Autodesk Inventor part; units mm, degrees
ref_plane "YZ Plane" through (0, 0, 0) normal (1, 0, 0) x (0, 1, 0)
ref_plane "XZ Plane" through (0, 0, 0) normal (0, 1, 0) x (-1, 0, 0)
ref_plane "XY Plane" through (0, 0, 0) normal (0, 0, 1) x (1, 0, 0)
sketch "Sketch1" plane through (0, 0, 0) normal (1, 0, 0) x (0, 1, 0)
  line L0 (0, 0) -> (5.55, 0)
  line L1 (5.55, 0) -> (5.55, 5.6)
  line L2 (5.55, 5.6) -> (20.55, 5.6)
  line L3 (20.55, 5.6) -> (20.55, 2.4)
  line L4 (20.55, 2.4) -> (10.05, 2.4)
  line L5 (10.05, 2.4) -> (10.05, 4)
  line L6 (10.05, 4) -> (7.55, 4)
  line L7 (7.55, 4) -> (7.55, -29)
  line L8 (0, 0) -> (0, -29)
  line L9 (0, -29) -> (7.55, -29)
  dimension "d1" = 5.55
  dimension "d2" = 15
  dimension "d3" = 2
  dimension "d4" = 2.5
  dimension "d5" = 1.6
  dimension "d6" = 29
  dimension "d7" = 33
  dimension "d8" = 3.2
extrude "Extrusion1" add sketch "Sketch1" along normal blind 18
sketch "Sketch2" plane through (0, 10.05, 2.4) normal (0, 0, -1) x (-1, 0, 0)
  line L0 (0, 0) -> (-18, 0)
  line L1 (-9, 0) -> (-9, -5.1044) construction
  line L2 (-13, 2.82) -> (-5, 2.82)
  line L3 (-5, 2.82) -> (-5, -0.28)
  line L4 (-5, -0.28) -> (-13, -0.28)
  line L5 (-13, -0.28) -> (-13, 2.82)
  point P0 (0, -10.05)
  point P1 (-9, -0.28)
  dimension "d11" = 3.1
  dimension "d12" = 8
extrude "Extrusion2" cut sketch "Sketch2" against normal up to surface (3.2 mm away)
chamfer "Chamfer1" distance 1.2 angle 45 2 edges at (5, 9.77, 4.8) (13, 9.77, 4.8)
chamfer "Chamfer2" distance 1.6 angle 45 2 edges at (15.04, 10.05, 2.4) (2.96, 10.05, 2.4)
fillet "Fillet1" radius 1 4 edges at (9, 5.55, 5.6) (9, 20.55, 5.6) (18, 13.05, 5.6) (0, 13.05, 5.6)
sketch "Sketch3" plane through (0, 0, -29) normal (0, 0, -1) x (-1, 0, 0)
  line L0 (0, 7.55) -> (-18, 7.55)
  line L1 (-9, 7.55) -> (-9, 5.1292) construction
  line L2 (-18, 7.55) -> (-15, 7.55)
  line L3 (-15, 7.55) -> (-15, 5.95)
  line L4 (-15, 5.95) -> (-18, 5.95)
  line L5 (-18, 5.95) -> (-18, 7.55)
  line L6 (0, 7.55) -> (-3, 7.55)
  line L7 (-3, 7.55) -> (-3, 5.95)
  line L8 (-3, 5.95) -> (0, 5.95)
  line L9 (0, 5.95) -> (0, 7.55)
  line L10 (0, 7.55) -> (-18, 7.55)
  line L11 (-18, 0) -> (-18, 7.55)
  point P0 (0, 0)
  dimension "d22" = 3
  dimension "d23" = 1.6
extrude "Extrusion3" cut sketch "Sketch3" against normal up to surface (33 mm away)
chamfer "Chamfer3" distance 1.6 angle 45 2 edges at (16.5, 5.95, 4) (1.5, 5.95, 4)
sketch "Sketch4" plane through (0, 0, 0) normal (-1, 0, 0) x (0, 0, 1)
  line L0 (-17, 0) -> (-7, 0)
  line L1 (-7, 0) -> (-7, 16.55)
  line L2 (-7, 16.55) -> (-17, 16.55)
  line L3 (-17, 16.55) -> (-17, 0)
  line L4 (2.4, 5.95) -> (-29, 5.95)
  line L5 (-29, 0) -> (0, 0)
  line L6 (0, 0) -> (0, 5.55)
  line L7 (4.6, 20.55) -> (2.4, 20.55)
  dimension "d29" = 10
  dimension "d30" = 7
  dimension "d31" = 4
extrude "Extrusion4" add sketch "Sketch4" along normal blind 5
sketch "Sketch5" plane through (0, 16.55, -7) normal (0, 1, 0) x (1, 0, 0)
  line L0 (0, -9.4) -> (18, -9.4)
  line L1 (0, 0) -> (-5, 0)
  line L2 (0, 0) -> (0, 10)
  line L3 (0, 10) -> (-5, 10)
  line L4 (-5, 0) -> (-5, 10)
  line L5 (0, 10) -> (0, 22)
  line L6 (-5, 10) -> (-5, 0)
  line L7 (0, 10) -> (-5, 10)
  line L8 (-5, 10) -> (-5, 0)
  line L9 (-5, 0) -> (0, 0)
  line L10 (13, -9.4) -> (5, -9.4)
  line L11 (13, -9.4) -> (18, -9.4)
  line L12 (5, -9.4) -> (18, -9.4)
  line L13 (18, -9.4) -> (0, 10)
  line L14 (3, -9.4) -> (0, -9.4)
  line L15 (0, 0) -> (0, -9.4)
  line L16 (0, -9.4) -> (18, -9.4)
  point P0 (0, -7)
extrude "Extrusion5" add sketch "Sketch5" against normal blind 2.5
chamfer "Chamfer4" distance 1.35 angle 45 3 edges at (-5, 8.275, -7) (-5, 8.275, -17) (0, 2.975, -17)
properties part number "pro_micro_mount"
Geometry: final body of the model. Coordinates: model frame, mm. A direction names the side the tool comes from. Round coordinates to 2 decimals unless told otherwise and drop trailing zeros. Write each loop counter-clockwise with the first axis right and the second up, starting at its lowest first coordinate (ties: lowest second). Pieces come first, ordered by that corner, then holes.
Item 1: Section query D-D (z = -5). Return loops of the section in (x, y), plus the area to 3 significant figures.
Item 2: Mould query, pull axis X, two halves, no side actions, for faces 4 (the face through (9, 9.77, 5)), 5 (the face through (-0.68, 2.93, -17.67)), 6 (the face through (15, 7, -13)). Classes: +X half, -X half, draft (parallel to the pull), parting line (faces both ways), or undercut.
Item 3: Section query B-B (x = 8). Return loops of the section in (y, z), plus the area to 3 significant figures.
Item 4: Section query A-A (z = -19.5). Return loops of the section in (x, y).
Item 5: Set-up query: faces 1 (the face through (0, 10, -12)), 2 (the face through (9, 19, 2.4)), 3 (the face through (13, 12, 4)). Return all of +Z, -Z, +X, -X, +Y, -Y with unobstructed straight access to the full face (end or side cutting, diameter ignored); none if empty.
Item 6: Pin query (flat end, axial travel): P1, Ø1, axis at x = 10.5, y = 9, coming from the -Z side; P2, Ø1, axis at y = 18, z = -3, coming from the +X side; P3, Ø4, axis at y = 8, z = -10.5, coming from the +X side; P4, Ø3.5, axis at x = 9.5, z = -13.5, coming from the +Y side. Return the tip coordinate at first contact, or that it passes through.
Item 7: Material intervals for L1, parallel to X at y = 7.5, z = -11; L2, parallel to Y at x = 0.25, z = -11.5; L3, parallel to Y at x = 7.25, z = -3.5, sorted ascending.
Item 8: Section query C-C (y = 3). Return loops of the section in (x, z), plus the area to 3 significant figures.
Completed:
1. outline: (0, 0) - (18, 0) - (18, 5.95) - (15, 5.95) - (15, 7.55) - (3, 7.55) - (3, 5.95) - (0, 5.95) - close; (0, 14.05) - (11.13, 14.05) - (11.13, 16.55) - (0, 16.55) - close
1. area: 154 mm2
2. face 4: undercut
2. face 5: -X half
2. face 6: +X half
3. outline: (0, -29) - (7.55, -29) - (7.55, 4) - (9.77, 4) - (9.77, 5.6) - (6.55, 5.6) arc R1 ccw to (5.55, 4.6) - (5.55, 0) - (0, 0) - close; (12.87, 2.4) - (14.05, 2.4) - (14.05, -8.38) - (16.55, -8.38) - (16.55, 2.4) - (20.55, 2.4) - (20.55, 4.6) arc R1 ccw to (19.55, 5.6) - (12.87, 5.6) - close
3. area: 285 mm2
4. outline: (0, 0) - (18, 0) - (18, 5.95) - (15, 5.95) - (15, 7.55) - (3, 7.55) - (3, 5.95) - (0, 5.95) - close
5. face 1: -Z
5. face 2: -Z, +X, -X, +Y
5. face 3: +Z, -Z
6. P1: stops at z = 4
6. P2: passes through
6. P3: stops at x = 15
6. P4: stops at y = 7.55
7. L1: x = -5 to 0, 3 to 15
7. L2: y = 0 to 5.95, 14.05 to 16.55
7. L3: y = 0 to 7.55, 14.05 to 16.55
8. outline: (-5, -15.65) - (-3.65, -17) - (-1.35, -17) - (0, -18.35) - (0, -29) - (18, -29) - (18, 0) - (0, 0) - (0, -7) - (-3.65, -7) - (-5, -8.35) - close
8. area: 571 mm2
